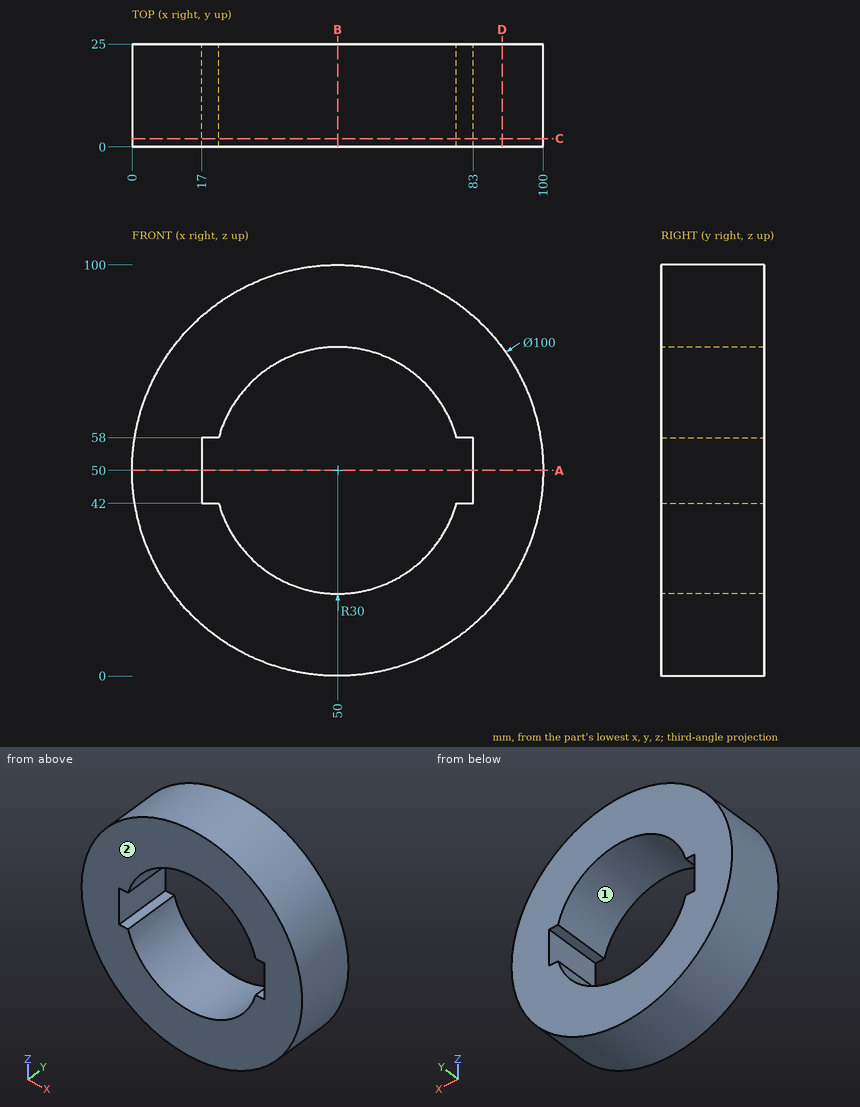
Can you work these out from the drawing? Everything is in mm from the part's minimum corner. A direction names the side the tool comes from. Give positions to 0.01 mm unless a question says otherwise; leave off trailing zeros. Loops run counter-clockwise (first coordinate to the right, second up) from the corner with the lowest first, then second, coordinate; pieces in that order, holes last. Notation, with made-up numbers: (47, 14) -> (98, 14) arc R24 ccw to (98, 28) -> close; hole circle Ø9 at (82.5, 28.5). An arc over 180 degrees is marked (long way). Return JSON: item names as keys, results as strings.
Q1. I want a section at B-B, the plane x = 50. List the corners of the cut face in (y, z) for me, then the cut area to 3 significant figures.
Checks:
{"outline": "(0, 0) -> (25, 0) -> (25, 20) -> (0, 20) -> close; (0, 80) -> (25, 80) -> (25, 100) -> (0, 100) -> close", "area": "1,000 mm2"}
Q2. I want a section at C-C, the plane y = 2. List the corners of the cut face in (x, z) for me.
Checks:
{"outline": "circle Ø100 at (50, 50); hole (17, 42) -> (21.09, 42) arc R30 ccw to (78.91, 42) -> (83, 42) -> (83, 58) -> (78.91, 58) arc R30 ccw to (21.09, 58) -> (17, 58) -> close"}
Q3. I want a section at A-A, the plane z = 50. List the corners of the cut face in (x, y) for me, then the cut area to 3 significant figures.
Checks:
{"outline": "(0, 0) -> (17, 0) -> (17, 25) -> (0, 25) -> close; (83, 0) -> (100, 0) -> (100, 25) -> (83, 25) -> close", "area": "850 mm2"}
Q4. On a 3-axis mill with a long thin cutter (end or side, diameter ignored), from which of +Z, -Z, +X, -X, +Y, -Y can I reach the whole of each face in a straight line? I mean the marked faces 1 and 2. Say none if no direction works.
Checks:
{"face 1": "+Y, -Y", "face 2": "+Z, -Z, +X, -X, -Y"}
Q5. I need wall thicknesses on probe 1 along Z at (x, y) = (80.5, 11.5); probe 2 along Z at (x, y) = (44.5, 4); probe 3 along X at (y, z) = (22.25, 77). Which ranges of each line are inside material? Lowest first, please.
Checks:
{"probe 1": "z = 10.38 to 42, 58 to 89.62", "probe 2": "z = 0.3 to 20.51, 79.49 to 99.7", "probe 3": "x = 7.92 to 36.92, 63.08 to 92.08"}
Q6. For pin 1 Ø13 at (y, z) = (7, 47.5) entering from +X; pin 2 Ø4.5 at (x, y) = (19, 9.5) entering from -Z; pin 3 Ø5 at (x, y) = (61.5, 13.5) entering from -Z; pin 4 Ø1.5 at (x, y) = (44, 9.5) entering from -Z, each with a flat end and sliding along its axis, tell me the tip position at first contact or that it passes through.
Checks:
{"pin 1": "stops at x = 100", "pin 2": "stops at z = 9.09", "pin 3": "stops at z = 0.82", "pin 4": "stops at z = 0.28"}
Q7. I want a section at D-D, the plane x = 90. List the corners of the cut face in (y, z) for me.
Checks:
{"outline": "(0, 20) -> (25, 20) -> (25, 80) -> (0, 80) -> close"}
